Autodesk Inventor part; units mm, degrees
ref_plane "YZ Plane" through (0, 0, 0) normal (1, 0, 0) x (0, 1, 0)
ref_plane "XZ Plane" through (0, 0, 0) normal (0, 1, 0) x (-1, 0, 0)
ref_plane "XY Plane" through (0, 0, 0) normal (0, 0, 1) x (1, 0, 0)
sketch "Sketch1" plane through (0, 0, 0) normal (0, 0, 1) x (1, 0, 0)
  line L0 (0, 0) -> (24.7, 0) construction
  line L1 (0, 105.5) -> (3, 105.5)
  line L2 (3, 142.5) -> (19, 142.5)
  line L3 (3, 142.5) -> (3, 105.5)
  line L4 (19, 142.5) -> (19, 95)
  line L5 (24.7, 81) -> (24.7, 0) construction
  line L6 (19, 95) -> (24.7, 95)
  line L7 (24.7, 95) -> (24.7, 81)
  line L8 (24.7, 81) -> (12.35, 81)
  line L9 (12.35, 81) -> (12.35, 75)
  line L10 (12.35, 75) -> (0, 75)
  line L11 (0, 75) -> (0, 0) construction
  line L12 (0, 105.5) -> (0, 75)
  dimension "d0" = 211
  dimension "d1" = 285
  dimension "d2" = 190
  dimension "d7" = 162
  dimension "d8" = 150
  dimension "d9" = 19
  dimension "d10" = 3
  dimension "d12" = 12.35
  dimension "d13" = 24.7
revolve "Revolution1" add sketch "Sketch1" angle 360 about axis through (0, 0, 0) along (1, 0, 0)
sketch "Sketch2" plane through (3, 0, 0) normal (-1, 0, 0) x (0, 0, 1)
  circle A0 centre (0, 0) radius 105.5
  line L0 (0, 0) -> (0, 120) construction
  circle A1 centre (0, 0) radius 142.5
  circle A2 centre (0, 0) radius 120 construction
  line L1 (0, 0) -> (45.922, 110.8655) construction
  circle A3 centre (45.922, 110.8655) radius 11.5
  dimension "d14" = 23
  dimension "d15" = 120
  dimension "d16" = 22.5
extrude "Extrusion1" cut sketch "Sketch2" against normal blind 19 contours A3
pattern_circular "Circular Pattern1" count 8 over 360 about axis through (1.5, 0, 0) along (1, 0, 0) of "Extrusion1"
equation "\"d0\" = D1"
equation "\"d1\" = D"
equation "\"d2\" = N3"
equation "\"d7\" = ID + 2 * t"
equation "\"d8\" = ID"
equation "\"d9\" = C1"
equation "\"d10\" = F1"
equation "\"d12\" = 0.65 * C1"
equation "\"d13\" = 1.3 * C1"
equation "\"d14\" = L"
equation "\"d15\" = 0.5 * K1"
equation "\"d3\" = C1"
equation "\"C1\" = 19"
equation "\"D\" = 285"
equation "\"L\" = 23"
equation "\"N3\" = 190"
equation "\"D1\" = 211"
equation "\"H1\" = 17"
equation "\"F1\" = 3"
equation "\"ID\" = 150"
equation "\"t\" = 6"
equation "\"Size_Designation\" = 1.2345"
properties part number "DIN EN 1092-2 Hubbed Socket Welding Flange Type 14 - PN 16 Ductile Iron DN150" material "Iron, Ductile"
Read the model definition and answer for the solid it produces. Units are mm, in the model's axes. A direction names the side the tool comes from. Coordinates: 2 decimals unless noted, no trailing zeros. Order: outer loops, then holes, each group sorted by start corner. A loop starts at its lowest first (then second) coordinate and runs counter-clockwise, first axis right, second up. Notation, with made-up numbers: (-7, -15.75) - (11, -15.75) arc R17 cw to (11, -3.75) - close; hole circle Ø1 at (31.5, -37). An arc over 180 degrees is marked (long way). Use one line per item in the form item = value.
(1) Which of the six approach directions +Z, -Z, +X, -X, +Y, -Y give full straight-line access (tool end or side, diameter ignored) to faces 5 (the face through (6.089, -9.764, -74.362)), 6 (the face through (21.89, -20.59, -92.74)), 7 (the face through (3, -1, 106))?
Computed values:
face_5 = +X, -X
face_6 = +X
face_7 = -X
(2) Given pin 1 Ø14 at (y, z) = (-110.87, 45.92) entering from -X; pin 2 Ø5 at (x, z) = (14.5, 14) entering from -Y; pin 3 Ø6 at (x, y) = (6, -47.5) entering from -Z; pin 4 Ø2 at (x, y) = (16.5, 12) entering from -Z, each flat-ended and moving along its own axis, determine where each tip first touches the part or whether it passes through.
Computed values:
pin_1 = through
pin_2 = -142.04
pin_3 = -135.37
pin_4 = -142.07
(3) Straight lines are drawn through the part: L1, parallel to Y at x = 12.5, z = 37.5; L2, parallel to Z at x = 8.5, y = 108.5; L3, parallel to Y at x = 14, z = -108. For each, find the intervals that lie inside material, in ascending order.
Computed values:
L1 = -137.48 to -118.7, -103.03 to -71.8, 71.8 to 103.03, 118.7 to 137.48
L2 = -92.38 to -57.18, -34.67 to 34.67, 57.18 to 92.38
L3 = -92.96 to -57.06, -34.78 to 34.78, 57.06 to 92.96
(4) Section C-C, the plane x = 15.75 is taken. Give the number of separate pieces and of enclosed holes in the cut face, then the cut area to 3 significant figures.
Computed values:
separate_pieces = 1
enclosed_holes = 9
area = 39,900 mm²
(5) For a pull along Y with two mould halves and no side action, classify faces 1 (the face through (10.89, -101.16, 39.75)), 2 (the face through (11.112, -105.028, 96.308)), 3 (the face through (10.888, -122.268, -44.425)), 4 (the face through (19, 93, -30)) as pulls with the +Y half, pulls with the -Y half, needs draft (parallel to the pull), parting line crosses it, or undercut.
Computed values:
face_1 = undercut
face_2 = parting line crosses it
face_3 = undercut
face_4 = needs draft
(6) Section D-D, the plane z = 85 is taken. Give the vertices of the cut face in (x, y).
Computed values:
outline = (0, -62.49) - (3, -62.49) - (3, -114.37) - (19, -114.37) - (19, -42.43) - (24.7, -42.43) - (24.7, 42.43) - (19, 42.43) - (19, 114.37) - (3, 114.37) - (3, 62.49) - (0, 62.49) - close
(7) Section A-A, the plane y = 0 is taken. Give the vertices of the cut face in (x, z).
Computed values:
outline = (0, -105.5) - (3, -105.5) - (3, -142.5) - (19, -142.5) - (19, -95) - (24.7, -95) - (24.7, -81) - (12.35, -81) - (12.35, -75) - (0, -75) - close; (0, 75) - (12.35, 75) - (12.35, 81) - (24.7, 81) - (24.7, 95) - (19, 95) - (19, 142.5) - (3, 142.5) - (3, 105.5) - (0, 105.5) - close
